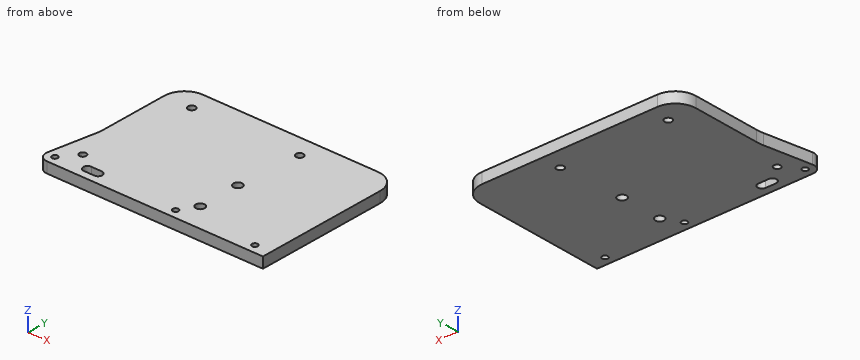
```python
from build123d import *

# Parameters (mm, degrees)
SKETCH1_R           = 2.1
SKETCH1_R_2         = 1.75
SKETCH1_R_3         = 1.35
SKETCH1_R_4         = 1.6
BOSS_EXTRUDE1_DEPTH = 5


with BuildPart() as part:
    # Sketch1 → Boss-Extrude1 (new body)
    with BuildSketch(Plane.XY):
        with BuildLine():
            Line((-62.05384494, 14.663645746), (-65.886192563, -7.070677654))
            ThreePointArc((-65.886192563, -7.070677654), (-64.967386661, -10.499707961), (-61.75, -12))
            Line((-61.75, -12), (40.25, -12))
            Line((40.25, -12), (40.25, 50.37))
            ThreePointArc((40.25, 50.37), (37.429438303, 57.179438303), (30.62, 60))
            Line((30.62, 60), (-52.12, 60))
            ThreePointArc((-52.12, 60), (-58.929438303, 57.179438303), (-61.75, 50.37))
            Line((-61.75, 50.37), (-61.75, 18.1366093))
            ThreePointArc((-61.75, 18.1366093), (-61.826106038, 16.393494445), (-62.05384494, 14.663645746))
        make_face()
        Circle(SKETCH1_R, mode=Mode.SUBTRACT)
        with Locations((-48.75, 50.37)):
            Circle(SKETCH1_R_2, mode=Mode.SUBTRACT)
        with Locations((32.75, -7.8)):
            Circle(SKETCH1_R_3, mode=Mode.SUBTRACT)
        with Locations(Location((2.25, 50.37, 0), (0, 0, 180))):
            Circle(SKETCH1_R_2, mode=Mode.SUBTRACT)
        with Locations((-61.75, -7.8)):
            Circle(SKETCH1_R_3, mode=Mode.SUBTRACT)
        with Locations((-4.75, -7.8)):
            Circle(SKETCH1_R_3, mode=Mode.SUBTRACT)
        with Locations((0, 20)):
            Circle(SKETCH1_R, mode=Mode.SUBTRACT)
        with Locations((-55.5, 0)):
            Circle(SKETCH1_R_4, mode=Mode.SUBTRACT)
        with BuildLine():
            Line((-47.5, -4.5), (-42.5, -4.5))
            ThreePointArc((-42.5, -4.5), (-40.5, -6.5), (-42.5, -8.5))
            Line((-42.5, -8.5), (-47.5, -8.5))
            ThreePointArc((-47.5, -8.5), (-49.5, -6.5), (-47.5, -4.5))
        make_face(mode=Mode.SUBTRACT)
    extrude(amount=BOSS_EXTRUDE1_DEPTH)


solid = part.part
```
Check sheet for the modelled part. Datum: model origin and axes. Units: mm. Coordinates: 2 decimals unless noted, no trailing zeros. Write each loop counter-clockwise with the first axis right and the second up, starting at its lowest first coordinate (ties: lowest second). Pieces come first, ordered by that corner, then holes. Notation, with made-up numbers: M 51,74 L 57,74 A19 ccw 57,86 Z; hole C 9.25,10.5 d8. An arc over 180 degrees is marked long. Use one line per item in the form item = value.
Item 1: Gauge pin test, flat end, axial feed: pin 1 Ø1 at (y, z) = (8.5, 3) entering from -X. Record the tip position at first contact, or that the pin passes through.
Answer below:
pin_1 = -63.23
Item 2: Sectioned sample at A-A, the plane y = 20. Record the cut outline in (x, z).
Answer below:
outline = M -61.75,0 L -2.1,0 L -2.1,5 L -61.75,5 Z; M 2.1,0 L 40.25,0 L 40.25,5 L 2.1,5 Z
Item 3: Material ranges on L1, parallel to Y at x = 0, z = 1.2; L2, parallel to X at y = 36.5, z = 0.8; L3, parallel to Y at x = 2.25, z = 1.5, recorded low to high. Write a range as from..to.
Answer below:
L1 = -12..-2.1, 2.1..17.9, 22.1..60
L2 = -61.75..40.25
L3 = -12..48.62, 52.12..60
Item 4: Sectioned sample at C-C, the plane z = 1.2. State how many separate pieces and enclosed holes the cut face has, and give its area (3 significant figures).
Answer below:
separate_pieces = 1
enclosed_holes = 9
area = 7,260 mm^2
Item 5: Sectioned sample at B-B, the plane x = -4.75. Record the cut outline in (y, z).
Answer below:
outline = M -12,0 L -9.15,0 L -9.15,5 L -12,5 Z; M -6.45,0 L 60,0 L 60,5 L -6.45,5 Z
Item 6: Sectioned sample at D-D, the plane y = 31. Record the cut outline in (x, z).
Answer below:
outline = M -61.75,0 L 40.25,0 L 40.25,5 L -61.75,5 Z
